from build123d import *

# Parameters (mm, degrees)
SKETCH1_W           = 65.5
SKETCH1_H           = 150
SKETCH1_R           = 2.75
BOSS_EXTRUDE1_DEPTH = 5
SKETCH2_R           = 6.5
BOSS_EXTRUDE2_DEPTH = 50
SKETCH3_R           = 7.5
BOSS_EXTRUDE3_DEPTH = 2
SKETCH4_R           = 1.65
SKETCH4_R_2         = 21.5
CUT_EXTRUDE1_DEPTH  = 100.732454597


with BuildPart() as part:
    # Sketch1 → Boss-Extrude1 (new body)
    with BuildSketch(Plane.XY):
        Rectangle(SKETCH1_W, SKETCH1_H)
        with Locations((-19.85, -62)):
            Circle(SKETCH1_R, mode=Mode.SUBTRACT)
        with Locations((19.85, -62)):
            Circle(SKETCH1_R, mode=Mode.SUBTRACT)
    extrude(amount=BOSS_EXTRUDE1_DEPTH)

    # Sketch2 → Boss-Extrude2 (add)
    with BuildSketch(Plane.XY.offset(5)):
        with Locations((0, 60)):
            Circle(SKETCH2_R)
    extrude(amount=BOSS_EXTRUDE2_DEPTH)

    # Sketch3 → Boss-Extrude3 (add)
    with BuildSketch(Plane.XY.offset(55)):
        with Locations((0, 60)):
            Circle(SKETCH3_R)
    extrude(amount=BOSS_EXTRUDE3_DEPTH)

    # Sketch4 → Cut-Extrude1 (cut, through all)
    with BuildSketch(Plane(origin=(0, 0, 0), x_dir=(-1, 0, 0), z_dir=(0, 0, -1))):
        with Locations((26.187094913, 17.5)):
            Circle(SKETCH4_R)
        with Locations((-8.812905087, 17.5)):
            Circle(SKETCH4_R)
        with Locations((-8.812905087, -17.5)):
            Circle(SKETCH4_R)
        with Locations((26.187094913, -17.5)):
            Circle(SKETCH4_R)
        with Locations((8.687094913, 0)):
            Circle(SKETCH4_R_2)
    extrude(amount=-CUT_EXTRUDE1_DEPTH, mode=Mode.SUBTRACT)


solid = part.part
Read the model definition and answer for the solid it produces. Units are mm, in the model's axes. A direction names the side the tool comes from. Round coordinates to 2 decimals unless told otherwise and drop trailing zeros. Write each loop counter-clockwise with the first axis right and the second up, starting at its lowest first coordinate (ties: lowest second). Pieces come first, ordered by that corner, then holes. Notation, with made-up numbers: M 1,-16.5 L 22,-16.5 A28 cw 22,11.5 Z; hole C -5.5,38.5 d1. An arc over 180 degrees is marked long. Use a Markdown table: item, result.
1) For a pull along X with two mould halves and no side action, classify faces 1 (the flat face through (14, 1, 0)), 2 (the flat face through (-32.75, -1, 2)), 3 (the cylindrical face through (-24.54, -17.43, 2.46)), 4 (the cylindrical face through (7.926, -16.109, 2.465)) as pulls with the +X half, pulls with the -X half, needs draft (parallel to the pull), parting line crosses it, or undercut.
Answers follow:
| item | result |
|---|---|
| face 1 | needs draft |
| face 2 | pulls with the -X half |
| face 3 | undercut |
| face 4 | undercut |
2) Straight lines are drawn through the part: line 1 along X through (y, z) = (-17, 1); line 2 along Z through (x, y) = (11.5, 56.5); line 3 along Y through (x, z) = (19, 4). For each, find the intervals that lie inside material, in ascending order. Write a range as [from, to].
Answers follow:
| item | result |
|---|---|
| line 1 | x = [-32.75, -27.76], [-24.61, -21.85], [4.48, 7.24], [10.39, 32.75] |
| line 2 | z = [0, 5] |
| line 3 | y = [-75, -64.62], [-59.38, 75] |
3) Flat-ended cylindrical pins translate along their axes: pin 1 (4 mm diameter, centred on x = -26.19, y = 17.5, fed in from +Z); pin 2 (1 mm diameter, centred on x = 2.5, z = 43, fed in from -Y); pin 3 (5 mm diameter, centred on x = -19.85, y = -62, fed in from -Z). Find the tip coordinate at first contact, or state that the pin passes through.
Answers follow:
| item | result |
|---|---|
| pin 1 | stops at z = 5 |
| pin 2 | stops at y = 53.82 |
| pin 3 | passes through |
4) A tool of negligible diameter and unlimited length cuts with its end or side. For faces 5 (the cylindrical face through (-20.208, -59.273, 2.465)), 6 (the cylindrical face through (-1.409, 53.655, 29.65)), 7 (the cylindrical face through (-0.976, 67.436, 55.986)), from which of +Z, -Z, +X, -X, +Y, -Y can it reach the whole face along a straight path? Write none if from no direction.
Answers follow:
| item | result |
|---|---|
| face 5 | +Z, -Z |
| face 6 | none |
| face 7 | +Z |
5) The part is cut by section D-D (y = -17.5). Write down the section's boundary in (x, z).
Answers follow:
| item | result |
|---|---|
| outline | M -32.75,0 L -27.84,0 L -27.84,5 L -32.75,5 Z; M -24.54,0 L -21.18,0 L -21.18,5 L -24.54,5 Z; M 3.8,0 L 7.16,0 L 7.16,5 L 3.8,5 Z; M 10.46,0 L 32.75,0 L 32.75,5 L 10.46,5 Z |
6) The part is cut by section A-A (y = -62). Write down the section's boundary in (x, z).
Answers follow:
| item | result |
|---|---|
| outline | M -32.75,0 L -22.6,0 L -22.6,5 L -32.75,5 Z; M -17.1,0 L 17.1,0 L 17.1,5 L -17.1,5 Z; M 22.6,0 L 32.75,0 L 32.75,5 L 22.6,5 Z |
7) The part is cut by section B-B (y = 0). Write down the section's boundary in (x, z).
Answers follow:
| item | result |
|---|---|
| outline | M -32.75,0 L -30.19,0 L -30.19,5 L -32.75,5 Z; M 12.81,0 L 32.75,0 L 32.75,5 L 12.81,5 Z |
8) The part is cut by section C-C (x = 19.5). Write down the section's boundary in (y, z).
Answers follow:
| item | result |
|---|---|
| outline | M -75,0 L -64.73,0 L -64.73,5 L -75,5 Z; M -59.27,0 L 75,0 L 75,5 L -59.27,5 Z |
